from build123d import *

# Parameters (mm, degrees)
SKETCH1_W           = 260
SKETCH1_H           = 270
BOSS_EXTRUDE1_DEPTH = 6
SKETCH2_W           = 20
SKETCH2_H           = 6
CUT_EXTRUDE1_DEPTH  = 6
CUT_EXTRUDE2_DEPTH  = 10
SKETCH4_W           = 6
SKETCH4_H           = 44.5
SKETCH4_H_2         = 15
SKETCH4_H_3         = 36
CUT_EXTRUDE3_DEPTH  = 6
SKETCH5_R           = 8
CUT_EXTRUDE4_DEPTH  = 10
SKETCH6_R           = 1.55
CUT_EXTRUDE5_DEPTH  = 6
CUT_EXTRUDE7_DEPTH  = 10
SKETCH8_W           = 248
SKETCH8_H           = 6
BOSS_EXTRUDE2_DEPTH = 5
BOSS_EXTRUDE3_DEPTH = 6
SKETCH10_W          = 6
SKETCH10_H          = 5
CUT_EXTRUDE8_DEPTH  = 6
SKETCH11_R          = 1.55
CUT_EXTRUDE9_DEPTH  = 6
SKETCH12_R          = 1.55
CUT_EXTRUDE10_DEPTH = 10
SKETCH13_W          = 269
SKETCH13_H          = 6
BOSS_EXTRUDE4_DEPTH = 14
SKETCH14_W          = 34
SKETCH14_H          = 6
SKETCH14_W_2        = 10.5
SKETCH14_W_3        = 44.5
BOSS_EXTRUDE5_DEPTH = 4
SKETCH15_R          = 1.55
SKETCH15_W          = 20
SKETCH15_H          = 6
CUT_EXTRUDE11_DEPTH = 10


with BuildPart() as part:
    # Sketch1 → Boss-Extrude1 (new body)
    with BuildSketch(Plane.XY):
        with Locations((130, 135)):
            Rectangle(SKETCH1_W, SKETCH1_H)
    extrude(amount=BOSS_EXTRUDE1_DEPTH)

    # Sketch2 → Cut-Extrude1 (cut)
    with BuildSketch(Plane(origin=(0, 0, 0), x_dir=(-1, 0, 0), z_dir=(0, 0, -1))):
        with Locations((-215, 53)):
            Rectangle(SKETCH2_W, SKETCH2_H)
        with Locations((-175, 53)):
            Rectangle(SKETCH2_W, SKETCH2_H)
        with BuildLine():
            Line((-220, 0), (-40, 0))
            ThreePointArc((-40, 0), (-130, 10), (-220, 0))
        make_face()
        with Locations((-85, 53)):
            Rectangle(SKETCH2_W, SKETCH2_H)
        with Locations((-45, 53)):
            Rectangle(SKETCH2_W, SKETCH2_H)
    extrude(amount=-CUT_EXTRUDE1_DEPTH, mode=Mode.SUBTRACT)

    # Sketch3 → Cut-Extrude2 (cut)
    with BuildSketch(Plane(origin=(0, 0, 0), x_dir=(-1, 0, 0), z_dir=(0, 0, -1))):
        with BuildLine():
            Line((-225, 70), (-35, 70))
            ThreePointArc((-35, 70), (-31.464466094, 71.464466094), (-30, 75))
            Line((-30, 75), (-30, 220))
            ThreePointArc((-30, 220), (-31.464466094, 223.535533906), (-35, 225))
            Line((-35, 225), (-225, 225))
            ThreePointArc((-225, 225), (-228.535533906, 223.535533906), (-230, 220))
            Line((-230, 220), (-230, 75))
            ThreePointArc((-230, 75), (-228.535533906, 71.464466094), (-225, 70))
        make_face()
    extrude(amount=-CUT_EXTRUDE2_DEPTH, mode=Mode.SUBTRACT)

    # Sketch4 → Cut-Extrude3 (cut)
    with BuildSketch(Plane(origin=(0, 0, 0), x_dir=(-1, 0, 0), z_dir=(0, 0, -1))):
        Polygon((-254, 270), (-260, 270), (-260, 264), (-260, 255), (-254, 255), (-254, 264), align=None)
        with Locations((-257, 212.75)):
            Rectangle(SKETCH4_W, SKETCH4_H)
        with Locations((-257, 163)):
            Rectangle(SKETCH4_W, SKETCH4_H_2)
        with Locations((-257, 113.25)):
            Rectangle(SKETCH4_W, SKETCH4_H)
        with Locations((-257, 53)):
            Rectangle(SKETCH4_W, SKETCH4_H_3)
        with Locations((-257, 7.5)):
            Rectangle(SKETCH4_W, SKETCH4_H_2)
        with Locations((-3, 7.5)):
            Rectangle(SKETCH4_W, SKETCH4_H_2)
        with Locations((-3, 53)):
            Rectangle(SKETCH4_W, SKETCH4_H_3)
        with Locations((-3, 113.25)):
            Rectangle(SKETCH4_W, SKETCH4_H)
        with Locations((-3, 212.75)):
            Rectangle(SKETCH4_W, SKETCH4_H)
        with Locations((-3, 262.5)):
            Rectangle(SKETCH4_W, SKETCH4_H_2)
        with Locations((-3, 163)):
            Rectangle(SKETCH4_W, SKETCH4_H_2)
    extrude(amount=-CUT_EXTRUDE3_DEPTH, mode=Mode.SUBTRACT)

    # Sketch5 → Cut-Extrude4 (cut)
    with BuildSketch(Plane(origin=(0, 0, 0), x_dir=(-1, 0, 0), z_dir=(0, 0, -1))):
        with Locations((-235, 240.5)):
            Circle(SKETCH5_R)
        with Locations((-25, 240.5)):
            Circle(SKETCH5_R)
    extrude(amount=-CUT_EXTRUDE4_DEPTH, mode=Mode.SUBTRACT)

    # Sketch6 → Cut-Extrude5 (cut)
    with BuildSketch(Plane.XY.offset(6)):
        with Locations((34.20128912, 249.683478563)):
            Circle(SKETCH6_R)
        with Locations((15.816521437, 231.29871088)):
            Circle(SKETCH6_R)
        with Locations(Location((225.79871088, 249.683478563, 0), (0, 0, 180))):
            Circle(SKETCH6_R)
        with Locations(Location((244.183478563, 231.29871088, 0), (0, 0, 180))):
            Circle(SKETCH6_R)
    extrude(amount=-CUT_EXTRUDE5_DEPTH, mode=Mode.SUBTRACT)

    # Sketch7 → Cut-Extrude7 (cut)
    with BuildSketch(Plane.XY.offset(6)):
        with BuildLine():
            Line((30, 225), (30, 202.90481405))
            Line((30, 202.90481405), (230, 202.90481405))
            Line((230, 202.90481405), (230, 225))
            ThreePointArc((230, 225), (229.021842565, 227.970653528), (226.470087046, 229.779000322))
            ThreePointArc((226.470087046, 229.779000322), (130, 244.281446445), (33.529912954, 229.779000322))
            ThreePointArc((33.529912954, 229.779000322), (30.978157435, 227.970653528), (30, 225))
        make_face()
    extrude(amount=-CUT_EXTRUDE7_DEPTH, mode=Mode.SUBTRACT)

    # Sketch8 → Boss-Extrude2 (add)
    with BuildSketch(Plane(origin=(0, 270, 0), x_dir=(1, 0, 0), z_dir=(0, 1, 0))):
        with Locations((130, -3)):
            Rectangle(SKETCH8_W, SKETCH8_H)
    extrude(amount=BOSS_EXTRUDE2_DEPTH)

    # Sketch9 → Boss-Extrude3 (add)
    with BuildSketch(Plane.XY.offset(6)):
        Polygon((0, 270), (0, 0), (-4.5, 0), (-4.5, 275), (6, 275), (6, 270), align=None)
        Polygon((264.5, 275), (264.5, 0), (260, 0), (260, 270), (254, 270), (254, 275), align=None)
    extrude(amount=-BOSS_EXTRUDE3_DEPTH)

    # Sketch10 → Cut-Extrude8 (cut)
    with BuildSketch(Plane.XY.offset(6)):
        with Locations((3, 272.5)):
            Rectangle(SKETCH10_W, SKETCH10_H)
        with Locations((257, 272.5)):
            Rectangle(SKETCH10_W, SKETCH10_H)
    extrude(amount=-CUT_EXTRUDE8_DEPTH, mode=Mode.SUBTRACT)

    # Sketch11 → Cut-Extrude9 (cut)
    with BuildSketch(Plane.XY.offset(6)):
        with Locations((3, 245)):
            Circle(SKETCH11_R)
        with Locations((3, 180.5)):
            Circle(SKETCH11_R)
        with Locations((3, 145.5)):
            Circle(SKETCH11_R)
        with Locations((3, 81)):
            Circle(SKETCH11_R)
        with Locations((3, 25)):
            Circle(SKETCH11_R)
        with Locations(Location((257, 25, 0), (0, 0, 180))):
            Circle(SKETCH11_R)
        with Locations(Location((257, 81, 0), (0, 0, 180))):
            Circle(SKETCH11_R)
        with Locations(Location((257, 145.5, 0), (0, 0, 180))):
            Circle(SKETCH11_R)
        with Locations(Location((257, 180.5, 0), (0, 0, 180))):
            Circle(SKETCH11_R)
        with Locations(Location((257, 245, 0), (0, 0, 180))):
            Circle(SKETCH11_R)
    extrude(amount=-CUT_EXTRUDE9_DEPTH, mode=Mode.SUBTRACT)

    # Sketch12 → Cut-Extrude10 (cut)
    with BuildSketch(Plane.XY.offset(6)):
        with Locations((25, 53)):
            Circle(SKETCH12_R)
        with Locations((65, 53)):
            Circle(SKETCH12_R)
        with Locations((155, 53)):
            Circle(SKETCH12_R)
        with Locations(Location((195, 53, 0), (0, 0, 180))):
            Circle(SKETCH12_R)
        with Locations(Location((235, 53, 0), (0, 0, 180))):
            Circle(SKETCH12_R)
        with Locations((105, 53)):
            Circle(SKETCH12_R)
    extrude(amount=-CUT_EXTRUDE10_DEPTH, mode=Mode.SUBTRACT)

    # Sketch13 → Boss-Extrude4 (add)
    with BuildSketch(Plane(origin=(0, 275, 0), x_dir=(1, 0, 0), z_dir=(0, 1, 0))):
        with Locations((130, -3)):
            Rectangle(SKETCH13_W, SKETCH13_H)
    extrude(amount=BOSS_EXTRUDE4_DEPTH)

    # Sketch14 → Boss-Extrude5 (add)
    with BuildSketch(Plane.XZ):
        with Locations((23, 3)):
            Rectangle(SKETCH14_W, SKETCH14_H)
        with Locations((0.75, 3)):
            Rectangle(SKETCH14_W_2, SKETCH14_H)
        with Locations((242.25, 3)):
            Rectangle(SKETCH14_W_3, SKETCH14_H)
    extrude(amount=BOSS_EXTRUDE5_DEPTH)

    # Sketch15 → Cut-Extrude11 (cut)
    with BuildSketch(Plane.XY.offset(6)):
        with Locations((25, 278)):
            Circle(SKETCH15_R)
        with Locations((105, 278)):
            Circle(SKETCH15_R)
        with Locations((65, 278)):
            Circle(SKETCH15_R)
        with Locations(Location((195, 278, 0), (0, 0, 180))):
            Circle(SKETCH15_R)
        with Locations(Location((155, 278, 0), (0, 0, 180))):
            Circle(SKETCH15_R)
        with Locations(Location((235, 278, 0), (0, 0, 180))):
            Circle(SKETCH15_R)
        with Locations((45, 278)):
            Rectangle(SKETCH15_W, SKETCH15_H)
        with Locations((85, 278)):
            Rectangle(SKETCH15_W, SKETCH15_H)
        with Locations((175, 278)):
            Rectangle(SKETCH15_W, SKETCH15_H)
        with Locations((215, 278)):
            Rectangle(SKETCH15_W, SKETCH15_H)
    extrude(amount=-CUT_EXTRUDE11_DEPTH, mode=Mode.SUBTRACT)


solid = part.part
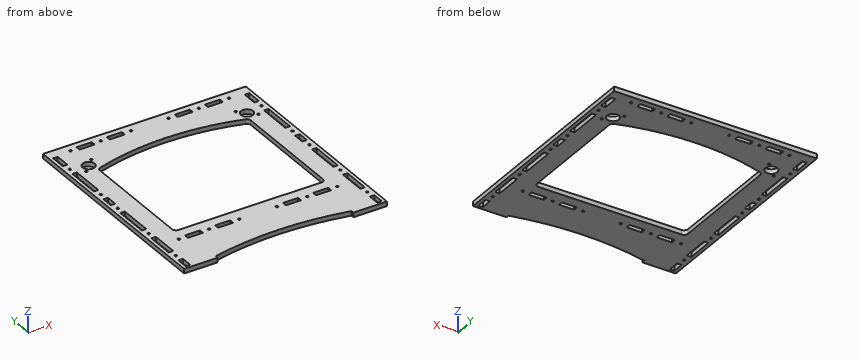
Part model, mm, in its own coordinate system. Round coordinates to 2 decimals unless told otherwise and drop trailing zeros. Write each loop counter-clockwise with the first axis right and the second up, starting at its lowest first coordinate (ties: lowest second). Pieces come first, ordered by that corner, then holes. Notation, with made-up numbers: M -27,4.25 L 28,4.25 A23 ccw 28,36.25 Z; hole C -9,66 d10. An arc over 180 degrees is marked long. Return JSON: item names as keys, results as strings. Group by question number.
(1) Drill centre lines: probe 1 along X at (y, z) = (249.5, 3.55); probe 2 along X at (y, z) = (126.5, 3.05); probe 3 along Y at (x, z) = (84.5, 4.55). Where is each one in solid material? Low to high.
(2) Saw through at B-B on y = 205.5. Write the cut outline in (x, z).
(3) Saw through at C-C on x = 79.5. Write the cut outline in (y, z), then the cut area to 4 significant figures.
(4) Saw through at D-D on z = 3.05. Count the separate pieces of the cut face and the enclosed holes in it, then the cut area to 3 significant figures.
(5) Pin check, flat tips, straight feed: pin 1 Ø5 at (x, y) = (3, 25) entering from +Z; pin 2 Ø1.8 at (x, z) = (217.5, 3.5) entering from -Y. Stop position of each tip, or through.
(6) Saw through at A-A on y = 268.5. Write the cut outline in (x, z).
Returned:
{
 "1": {"probe 1": "-4.5 to 32.66, 35.74 to 224.26, 227.34 to 264.5", "probe 2": "-4.5 to 0, 6 to 30, 230 to 254, 260 to 264.5", "probe 3": "7.47 to 50, 56 to 70, 241.11 to 275, 281 to 289"},
 "2": {"outline": "M -4.5,0 L 0,0 L 0,6 L -4.5,6 Z; M 6,0 L 30,0 L 30,6 L 6,6 Z; M 230,0 L 254,0 L 254,6 L 230,6 Z; M 260,0 L 264.5,0 L 264.5,6 L 260,6 Z"},
 "3": {"outline": "M 6.88,0 L 50,0 L 50,6 L 6.88,6 Z; M 56,0 L 70,0 L 70,6 L 56,6 Z; M 240.37,0 L 275,0 L 275,6 L 240.37,6 Z; M 281,0 L 289,0 L 289,6 L 281,6 Z", "area": "598.5 mm²"},
 "4": {"separate pieces": "1", "enclosed holes": "49", "area": "39,400 mm²"},
 "5": {"pin 1": "z = 6", "pin 2": "y = 0.36"},
 "6": {"outline": "M -4.5,0 L 0,0 L 0,6 L -4.5,6 Z; M 6,0 L 254,0 L 254,6 L 6,6 Z; M 260,0 L 264.5,0 L 264.5,6 L 260,6 Z"}
}
